Study the drawing (mm; zero at the part's minimum x, y, z) and answer. Give positions to 0.01 mm unless a question says otherwise; leave off trailing zeros. Loops run counter-clockwise (first coordinate to the right, second up) from the corner with the lowest first, then second, coordinate; pieces in that order, holes last. Notation, with made-up numbers: (-24, 88) - (-4, 88) arc R15 cw to (-4, 106) - close; hole circle Ø11 at (34.5, 43). An arc over 180 degrees is marked (long way). Write item = value, one per line. Start each with the question number.
1) The part is cut by section B-B on x = 250. Write down the section's boundary in (y, z), plus the area to 3 significant figures.
2) A flat-ended cylindrical pin translates along its axis: P1, Ø1, axis at x = 191.5, y = 172, coming from the -Z side. Find the tip coordinate at first contact, or state that the pin passes through.
3) Consider probe 1 along Y at (x, z) = (250, 4.5); probe 2 along Y at (x, z) = (270, 3). Determine where each line is inside the solid, lowest interval first.
4) The part is cut by section A-A on y = 100. Write down the section's boundary in (x, z), plus the area to 3 significant figures.
5) The part is cut by section C-C on z = 2. Write down the section's boundary in (x, y), plus the area to 3 significant figures.
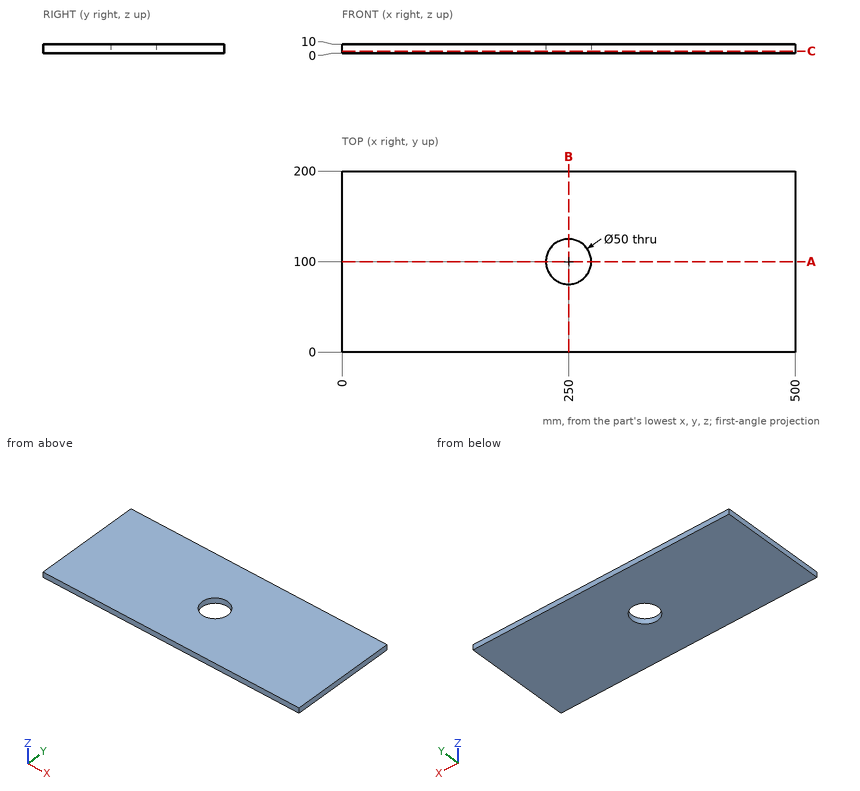
Answer below:
q1.outline = (0, 0) - (75, 0) - (75, 10) - (0, 10) - close; (125, 0) - (200, 0) - (200, 10) - (125, 10) - close
q1.area = 1,500 mm2
q2.P1 = 0
q3.probe_1 = 0 to 75, 125 to 200
q3.probe_2 = 0 to 85, 115 to 200
q4.outline = (0, 0) - (225, 0) - (225, 10) - (0, 10) - close; (275, 0) - (500, 0) - (500, 10) - (275, 10) - close
q4.area = 4,500 mm2
q5.outline = (0, 0) - (500, 0) - (500, 200) - (0, 200) - close; hole circle Ø50 at (250, 100)
q5.area = 98,000 mm2
